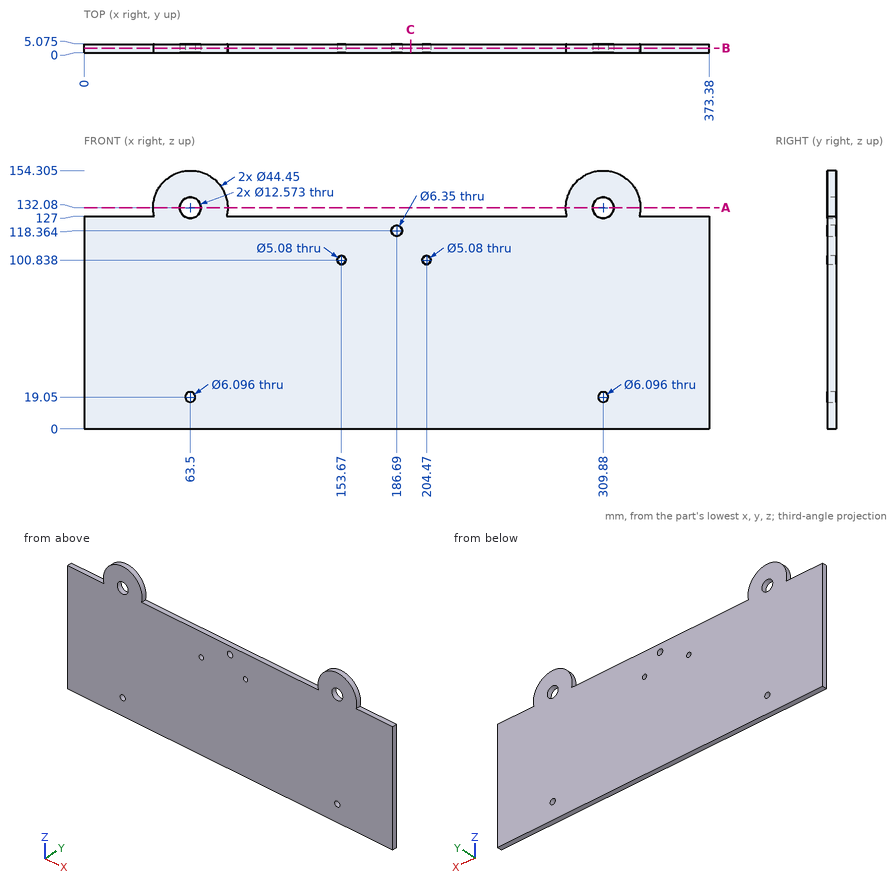
Drawing for the job (mm, zero at the part's lowest x, y, z). Give positions to 0.01 mm unless a question says otherwise; leave off trailing zeros. Loops run counter-clockwise (first coordinate to the right, second up) from the corner with the lowest first, then second, coordinate; pieces in that order, holes last. Notation, with made-up numbers: (-3, 85.5) - (17, 85.5) arc R23 ccw to (17, 95.5) - close; hole circle Ø5 at (55.25, 33). An arc over 180 degrees is marked (long way). Write item = value, one per line. Start each with the question number.
1) Band-saw the part on A-A on z = 132.08. Give the cut face in (x, y) (1 decimal).
2) Band-saw the part on B-B on y = 2.55. Count the separate pieces of the cut face and the enclosed holes in it, plus the area to 3 significant figures.
3) Probe probe 1 along X at (y, z) = (2.8, 19.05); probe 2 along Z at (x, y) = (309.88, 2.3) (1 decimal); probe 3 along X at (y, z) = (2.5, 132) (3 decimals). List the from-to ranges inside material, lowest first. Write a range as from..to.
4) Drop flat-ended pins along their axis: pin 1 Ø5 at (x, z) = (63.5, 19.05) entering from -Y; pin 2 Ø10 at (x, z) = (269.5, 125) entering from -Y; pin 3 Ø2.5 at (x, y) = (25.5, 2.5) entering from +Z. Give the stop position or say it passes through.
5) Band-saw the part on C-C on x = 195. Give the cut face in (y, z) (3 decimals).
Final values:
q1.outline = (41.3, 0) - (57.2, 0) - (57.2, 5.1) - (41.3, 5.1) - close; (69.8, 0) - (85.7, 0) - (85.7, 5.1) - (69.8, 5.1) - close; (287.7, 0) - (303.6, 0) - (303.6, 5.1) - (287.7, 5.1) - close; (316.2, 0) - (332.1, 0) - (332.1, 5.1) - (316.2, 5.1) - close
q2.separate_pieces = 1
q2.enclosed_holes = 7
q2.area = 49,000 mm²
q3.probe_1 = 0..60.45, 66.55..306.83, 312.93..373.38
q3.probe_2 = 0..16, 22.1..125.8, 138.4..154.3
q3.probe_3 = 41.275..57.214, 69.786..85.725, 287.655..303.594, 316.166..332.105
q4.pin_1 = through
q4.pin_2 = 0
q4.pin_3 = 127
q5.outline = (0, 0) - (5.075, 0) - (5.075, 127) - (0, 127) - close
